Check sheet for the modelled part. Datum: model origin and axes. Units: mm. A direction names the side the tool comes from. Round coordinates to 2 decimals unless told otherwise and drop trailing zeros. Write each loop counter-clockwise with the first axis right and the second up, starting at its lowest first coordinate (ties: lowest second). Pieces come first, ordered by that corner, then holes. Notation, with made-up numbers: M 80,55 L 98,55 A11 ccw 98,74 Z; hole C 58.25,-6 d10. An arc over 180 degrees is marked long. Answer in a Markdown table with one row per item.
```python
from build123d import *

# Parameters (mm, degrees)
F1_DEPTH = 50
F2_DEPTH = 20
F3_R     = 11.2180769553
F4_DEPTH = 64.881876111


with BuildPart() as f1:
    # F0 (on Front) → F1 (new body)
    with BuildSketch(Plane.XZ):
        with BuildLine():
            Line((-38.1, -25.4), (38.1, -25.4))
            Line((38.1, -25.4), (38.1, 25.4))
            Line((38.1, 25.4), (-38.1, 25.4))
            ThreePointArc((-38.1, 25.4), (-20.1394877579, 17.9605122421), (-12.7, 0))
            ThreePointArc((-12.7, 0), (-20.1394877579, -17.9605122421), (-38.1, -25.4))
        make_face()
        with BuildLine():
            ThreePointArc((-38.1, 25.4), (-63.5, 0), (-38.1, -25.4))
            Line((-38.1, -25.4), (-38.1, -19.05))
            ThreePointArc((-38.1, -19.05), (-57.15, 0), (-38.1, 19.05))
            Line((-38.1, 19.05), (-38.1, 25.4))
        make_face()
        with BuildLine():
            Line((-38.1, -19.05), (-38.1, -25.4))
            ThreePointArc((-38.1, -25.4), (-20.1394877579, -17.9605122421), (-12.7, 0))
            ThreePointArc((-12.7, 0), (-20.1394877579, 17.9605122421), (-38.1, 25.4))
            Line((-38.1, 25.4), (-38.1, 19.05))
            ThreePointArc((-38.1, 19.05), (-24.6296158184, 13.4703841816), (-19.05, 0))
            ThreePointArc((-19.05, 0), (-24.6296158184, -13.4703841816), (-38.1, -19.05))
        make_face()
    extrude(amount=F1_DEPTH)

    # F2 (add): a face of the model
    f2_faces = [f1.faces().sort_by_distance(p)[0] for p in [
        (0, -25, 25.4),
    ]]
    extrude(f2_faces, amount=F2_DEPTH)

    # F3 (on face) → F4 (join)
    with BuildSketch(Plane.XY.offset(45.4)):
        with Locations((11.7288976908, -29.2320102453)):
            Circle(F3_R)
    extrude(amount=F4_DEPTH)


solid = f1.part
```
1. Access from +Z, -Z, +X, -X, +Y, -Y to the whole of each face (thin tool, end or side, straight path). Record for faces 4 (the face through (10.27, -18.11, 77.39)), 5 (the face through (-63.494, -24.65, 0.559)).
Found:
| item | result |
|---|---|
| face 4 | +Z |
| face 5 | -X, +Y, -Y |
2. Section check C-C, the plane x = -25.5. Record the cut outline in (y, z).
Found:
| item | result |
|---|---|
| outline | M -50,-25.4 L 0,-25.4 L 0,-14.29 L -50,-14.29 Z; M -50,14.29 L 0,14.29 L 0,45.4 L -50,45.4 Z |
3. Section check D-D, the plane x = 31.5. Record the cut outline in (y, z), and give its area (3 significant figures).
Found:
| item | result |
|---|---|
| outline | M -50,-25.4 L 0,-25.4 L 0,45.4 L -50,45.4 Z |
| area | 3,540 mm2 |
4. Draft check along X on faces 1 (the face through (-57.13, -24.65, -0.84)), 2 (the face through (-1, 0, 10)), 3 (the face through (-38.1, -25, 35)). Enter one of: +X half, -X half, draft (parallel to the pull), parting line (faces both ways), or undercut.
Found:
| item | result |
|---|---|
| face 1 | undercut |
| face 2 | draft |
| face 3 | -X half |
5. Scan lines: L1, parallel to Z at x = -38, y = -23; L2, parallel to Z at x = -40.5, y = -20; L3, parallel to Z at x = -8, y = -32. Record each from-to range of solid material in increasing order.
Found:
| item | result |
|---|---|
| L1 | z = -25.4 to -19.05, 19.05 to 45.4 |
| L2 | z = -25.29 to -18.9, 18.9 to 25.29 |
| L3 | z = -25.4 to 45.4 |
6. Go/stop test with flat-tipped pins: pin 1 (16 mm diameter, centred on y = -33, z = 39, fed in from -X); pin 2 (12 mm diameter, centred on y = -37, z = 87.5, fed in from -X); pin 3 (3 mm diameter, centred on x = 28, y = -30, fed in from +Z). Record where each tip stops, or that it passes through.
Found:
| item | result |
|---|---|
| pin 1 | stops at x = -38.1 |
| pin 2 | stops at x = 0.65 |
| pin 3 | stops at z = 45.4 |
7. Section check A-A, the plane z = 0. Record the cut outline in (x, y), and give its area (4 significant figures).
Found:
| item | result |
|---|---|
| outline | M -63.5,-50 L -57.15,-50 L -57.15,0 L -63.5,0 Z; M -19.05,-50 L 38.1,-50 L 38.1,0 L -19.05,0 Z |
| area | 3,175 mm2 |
8. Section check B-B, the plane y = -5. Record the cut outline in (x, z), and give its area (3 significant figures).
Found:
| item | result |
|---|---|
| outline | M -38.1,-25.4 L 38.1,-25.4 L 38.1,45.4 L -38.1,45.4 L -38.1,25.4 A25.4 ccw Z; hole C -38.1,0 d38.1 |
| area | 5,270 mm2 |
